```python
from build123d import *

# Parameters (mm, degrees)
SKETCH_1_R      = 4.925
SKETCH_1_R_2    = 1.6
EXTRUDE_1_DEPTH = 8
FILLET_1_R      = 0.5


with BuildPart() as part:
    # 草图1 → 凸台-拉伸1 (new body)
    with BuildSketch(Plane(origin=(0, 0, 0), x_dir=(1, 0, 0), z_dir=(0, 1, 0))):
        with Locations(Location((0, 0, 0), (0, 0, 270))):
            Circle(SKETCH_1_R)
        with Locations(Location((0, 0, 0), (0, 0, 270))):
            Circle(SKETCH_1_R_2, mode=Mode.SUBTRACT)
    extrude(amount=EXTRUDE_1_DEPTH)

    # 圆角1
    fillet_1_edges = [part.edges().sort_by_distance(p)[0] for p in [
        (0, 0, -4.925),
        (0, 8, -4.925),
        (0, 0, -1.6),
    ]]
    fillet(fillet_1_edges, radius=FILLET_1_R)


solid = part.part
```
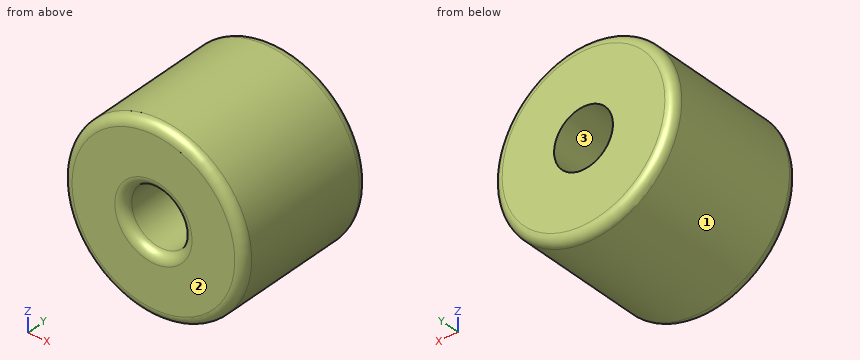
The listing builds one solid part. Answer for the finished solid, in the listing's coordinates (mm). Face numbers are marked on the shaded views. Coordinates: 2 decimals unless noted, no trailing zeros. Write each loop counter-clockwise with the first axis right and the second up, starting at its lowest first coordinate (ties: lowest second). Pieces come first, ordered by that corner, then holes. Notation, with made-up numbers: (13.25, 88) - (67.25, 88) arc R20 cw to (67.25, 115) - close; hole circle Ø3 at (-33, -19.5). An arc over 180 degrees is marked (long way). Return JSON: item names as keys, results as strings. Group by question number.
1. Determine the mould class of the marked faces 1, 2 and 3 for opening direction X: released by +X, released by -X, zero draft, split by the parting line, or undercut.
2. Straight lines are drawn through the part: L1, parallel to X at y = 6.25, z = 0 (3 decimals); L2, parallel to Z at x = 0.75, y = 7; L3, parallel to Z at x = -0.5, y = 4.5. For each, find the intervals that lie inside material, in ascending order.
3. Given pin 1 (4 mm diameter, centred on x = 0, z = 0, fed in from -Y); pin 2 (2 mm diameter, centred on x = -2, y = 2, fed in from +Z); pin 3 (2 mm diameter, centred on y = 1.5, z = -1.5, fed in from +X), each flat-ended and moving along its own axis, determine where each tip first touches the part or whether it passes through.
4. A cutting plane is placed at C-C, the plane y = 5.75. Determine the outline of the cut face in (x, z) (3 decimals), plus the area to 3 significant figures.
5. A cutting plane is placed at A-A, the plane z = 0. Determine the outline of the cut face in (x, y) (3 decimals).
6. A cutting plane is placed at B-B, the plane x = 0. Determine the outline of the cut face in (y, z) (3 decimals).
Ans:
{
 "1": {"face 1": "split by the parting line", "face 2": "zero draft", "face 3": "undercut"},
 "2": {"L1": "-4.925 to -1.6, 1.6 to 4.925", "L2": "-4.87 to -1.41, 1.41 to 4.87", "L3": "-4.9 to -1.52, 1.52 to 4.9"},
 "3": {"pin 1": "y = 0.01", "pin 2": "z = 4.82", "pin 3": "x = 4.9"},
 "4": {"outline": "circle Ø9.85 at (0, 0); hole circle Ø3.2 at (0, 0)", "area": "68.2 mm²"},
 "5": {"outline": "(-4.925, 0.5) arc R0.5 ccw to (-4.425, 0) - (-2.1, 0) arc R0.5 ccw to (-1.6, 0.5) - (-1.6, 8) - (-4.425, 8) arc R0.5 ccw to (-4.925, 7.5) - close; (1.6, 0.5) arc R0.5 ccw to (2.1, 0) - (4.425, 0) arc R0.5 ccw to (4.925, 0.5) - (4.925, 7.5) arc R0.5 ccw to (4.425, 8) - (1.6, 8) - close"},
 "6": {"outline": "(0, -4.425) arc R0.5 ccw to (0.5, -4.925) - (7.5, -4.925) arc R0.5 ccw to (8, -4.425) - (8, -1.6) - (0.5, -1.6) arc R0.5 ccw to (0, -2.1) - close; (0, 2.1) arc R0.5 ccw to (0.5, 1.6) - (8, 1.6) - (8, 4.425) arc R0.5 ccw to (7.5, 4.925) - (0.5, 4.925) arc R0.5 ccw to (0, 4.425) - close"}
}
